Answer from the drawing. Dimensions are ordinates in mm from the lowest x, y and z of the part. A direction names the side the tool comes from. Coordinates: 2 decimals unless noted, no trailing zeros. Order: outer loops, then holes, each group sorted by start corner. A loop starts at its lowest first (then second) coordinate and runs counter-clockwise, first axis right, second up. Notation, with made-up numbers: (24.25, 57) -> (56.25, 57) arc R30 cw to (56.25, 94) -> close; hole circle Ø10 at (82.25, 34). An arc over 180 degrees is marked (long way). Use CSV: the item, a comma, the result in double quotes.
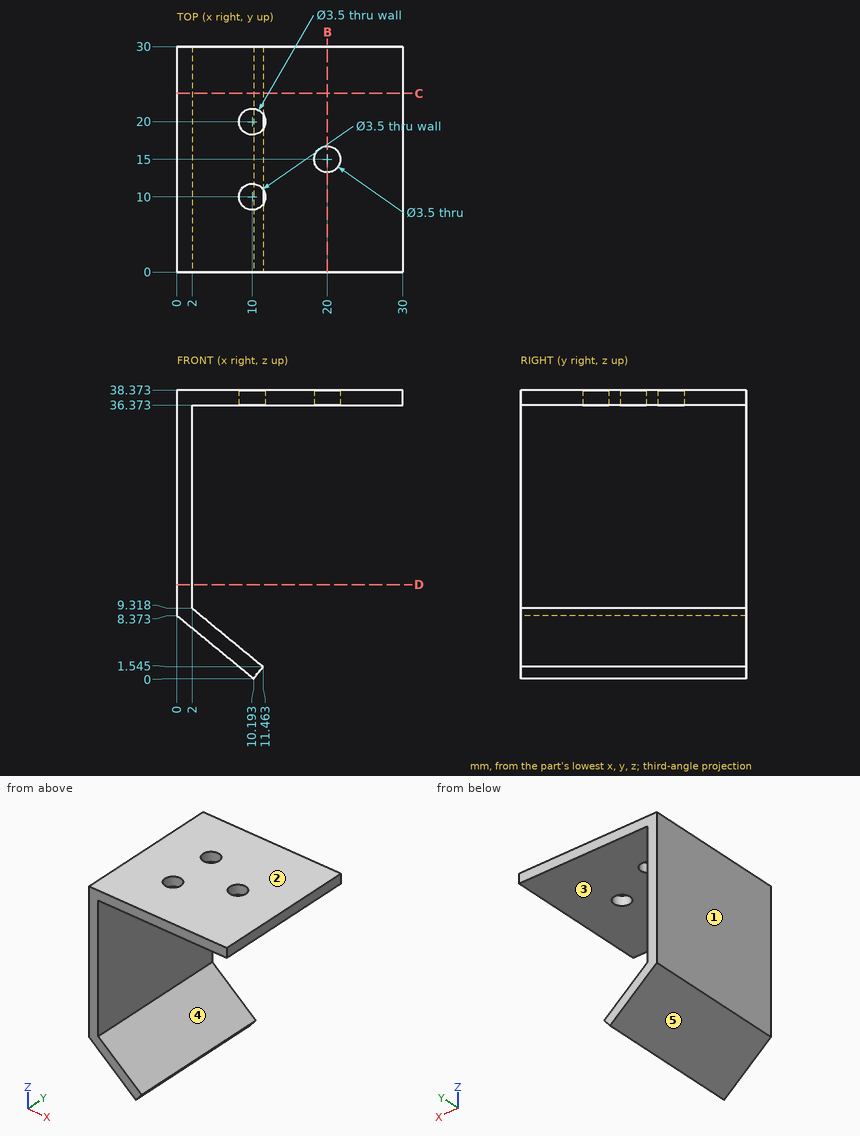
Item 1: The mould has two halves that part along Z. Classify the marked faces 1, 2 and 3: +Z half, -Z half, draft (parallel to the pull), parting line (faces both ways), or undercut.
Return value:
face 1,"draft"
face 2,"+Z half"
face 3,"undercut"
Item 2: Straight lines are drawn through the part: line 1 along Y through (x, z) = (10, 37.4); line 2 along Z through (x, y) = (15.25, 18.5); line 3 along X through (y, z) = (3.5, 26). For each, find the intervals that lie inside material, in ascending order.
Return value:
line 1,"y = 0 to 8.25, 11.75 to 18.25, 21.75 to 30"
line 2,"z = 36.37 to 38.37"
line 3,"x = 0 to 2"
Item 3: Each of these flat-tipped pins is pushed along its axis until it touches: P1, Ø3, axis at x = 10, y = 10, coming from the +Z side; P2, Ø6, axis at y = 24.5, z = 10.5, coming from the +X side (1 decimal); P3, Ø1.5, axis at y = 11.5, z = 5.5, coming from the +X side. Where does it stop, or does it pass through?
Return value:
P1,"stops at z = 3.98"
P2,"stops at x = 4.2"
P3,"stops at x = 7.56"
Item 4: Find section D-D, the plane z = 12.5. Give the vertices of the cut face in (x, y).
Return value:
outline,"(0, 0) -> (2, 0) -> (2, 30) -> (0, 30) -> close"
Item 5: A tool of negligible diameter and unlimited length cuts with its end or side. For the marked faces 4 and 5, from which of +Z, -Z, +X, -X, +Y, -Y can it reach the whole face along a straight path? Write none if from no direction.
Return value:
face 4,"+X, +Y, -Y"
face 5,"-Z, -X, +Y, -Y"
Item 6: Find section B-B, the plane x = 20. Give the vertices of the cut face in (y, z).
Return value:
outline,"(0, 36.37) -> (13.25, 36.37) -> (13.25, 38.37) -> (0, 38.37) -> close; (16.75, 36.37) -> (30, 36.37) -> (30, 38.37) -> (16.75, 38.37) -> close"
Item 7: Find section C-C, the plane y = 23.75. Give the vertices of the cut face in (x, z) (1 decimal).
Return value:
outline,"(0, 8.4) -> (10.2, 0) -> (11.5, 1.5) -> (2, 9.3) -> (2, 36.4) -> (30, 36.4) -> (30, 38.4) -> (0, 38.4) -> close"
